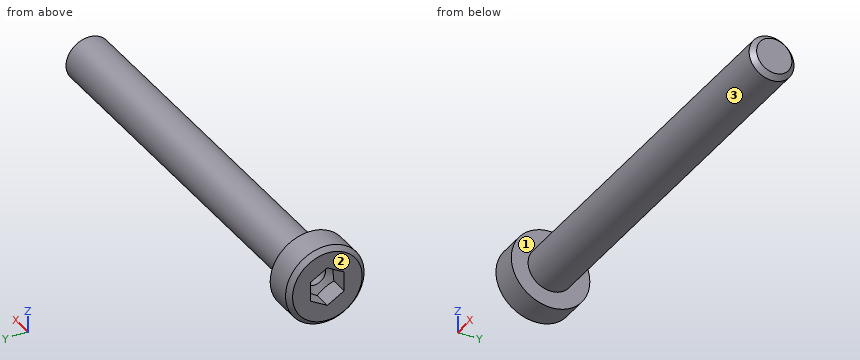
Autodesk Inventor part; units mm, degrees
ref_plane "Work Plane1" through (17.5, 0, 0) normal (0, 0.5, 0.866) x (1, 0, 0)
ref_plane "YZ Plane" through (0, 0, 0) normal (1, 0, 0) x (0, 1, 0)
ref_plane "XZ Plane" through (0, 0, 0) normal (0, 1, 0) x (-1, 0, 0)
sketch "Sketch1" plane through (0, 0, 0) normal (0, 0, 1) x (1, 0, 0)
  line L0 (1.0774, 0) -> (35, 0)
  line L1 (35, 0) -> (35, 2)
  line L2 (35, 2) -> (0, 2)
  line L3 (0, 2) -> (0, 3.5)
  line L4 (0, 3.5) -> (-2.8, 3.5)
  line L5 (-2.8, 3.5) -> (-2.8, 1.7321)
  line L6 (-2.8, 1.7321) -> (-1.2, 1.7321)
  line L7 (-1.2, 1.7321) -> (-0.7774, 1)
  line L8 (-10.36, 0) -> (42.56, 0)
  line L9 (0, -0.7) -> (0, 4.2)
  line L10 (-0.7774, 1) -> (0.5, 1)
  line L11 (0.5, 1) -> (1.0774, 0)
  line L12 (-2.8, 1.7321) -> (-2.8, 0) construction
  line L13 (-2.8, 3.1) -> (-2.4, 3.5)
  dimension "d0" = 2.8
  dimension "d1" = 1.6
  dimension "d2" = 60
  dimension "d3" = 4
  dimension "d4" = 3.4641
  dimension "d5" = 7
  dimension "d15" = 3.3
  dimension "d16" = 2
  dimension "d17" = 35
  dimension "d32" = 45
  dimension "d33" = 0.4
revolve "Body" add sketch "Sketch1" angle 360 about axis through (1.0774, 0, 0) along (1, 0, 0) contours L11 L10 L9 L2 L1 L0 | L10 L7 L6 L5 L13 L4 L3 L9 | L13 L5 L4
revolve "Chamfer2" cut sketch "Sketch1" angle 360 about axis through (-10, 0, 0) along (1, 0, 0) contours L13 L5 L4
sketch "Sketch2" plane through (-2.8, 0, 0) normal (-1, 0, 0) x (0, 0, 1)
  circle A0 centre (0, 0) radius 1.7321
  line L0 (0, -4.9) -> (0, 4.9)
  line L1 (-4.9, 0) -> (4.9, 0)
  line L2 (1.7321, 0) -> (0.866, -1.5)
  line L3 (0.866, -1.5) -> (-0.866, -1.5)
  line L4 (-0.866, -1.5) -> (-1.7321, 0)
  line L5 (-1.7321, 0) -> (-0.866, 1.5)
  line L6 (-0.866, 1.5) -> (0.866, 1.5)
  line L7 (0.866, 1.5) -> (1.7321, 0)
extrude "Slot" add sketch "Sketch2" against normal up to next contours L7 A0 | A0 L2 | L6 L0 A0 | A0 L0 L3 | L0 L6 A0 | A0 L3 L0 | L4 A0 | A0 L5
thread "Thread"
chamfer "Chamfer1" distance 0.4294 distance2 0.4294 1 edges at (35, -2, 0) measured on face at (35, 0.0262, -0.4421)
ref_plane "Work Plane1" through (17.5, 0, 0) normal (0, 0.5, 0.866) x (1, 0, 0)
equation "\"d0\" = KOH"
equation "\"d1\" = INTI"
equation "\"d3\" = GD"
equation "\"d4\" = 1.1547 * SW"
equation "\"d5\" = KOD"
equation "\"d15\" = INFT"
equation "\"d16\" = SDT"
equation "\"d17\" = NLG"
equation "\"d33\" = Cham"
equation "\"d7\" = GEL"
equation "\"d9\" = -0.5 * SPD + 0.5 * GD"
equation "\"d12\" = GUL"
equation "\"GD\" = NND"
equation "\"NLG\" = 35"
equation "\"GEL\" = 14"
equation "\"KOD\" = 7"
equation "\"KOH\" = 2.8"
equation "\"GUL\" = 0.61345 * PTC"
equation "\"SW\" = 3"
equation "\"INTI\" = 1.6"
equation "\"SPD\" = NND - 1.2269 * PTC"
equation "\"SDT\" = 2"
equation "\"INFT\" = 3.3"
equation "\"Cham\" = 0.4"
equation "\"TOA\" = 30deg"
equation "\"GD1\" = THREADDIA - 1.2269 * PTC"
equation "\"THREADDIA\" = 4"
equation "\"BDM\" = NND"
equation "\"FAWI\" = 45deg"
equation "\"RR\" = 0.1 * NND"
equation "\"PTC\" = 0.7"
equation "\"NND\" = 4"
equation "\"FAWI1\" = 45deg"
equation "\"GAL\" = 0.61345 * PTC"
equation "\"E0\" = 1.155 * SW"
properties part number "DIN 6912 - M4 x 35" material "Steel, Mild"
Design review of the part built by this model. Coordinates are the model's own, in mm. Face numbers are marked on the shaded views. Coordinates: 2 decimals unless noted, no trailing zeros. Loops run counter-clockwise (first coordinate to the right, second up) from the corner with the lowest first, then second, coordinate; pieces in that order, holes last.
Q1. To check wall thickness, follow line 1 (Z direction, x = 0.2, y = 0); line 2 (Z direction, x = -0.2, y = 0); line 3 (Z direction, x = 7.5, y = 0). State the ranges of each line that lie inside material, in increasing order.
Reported:
line 1: z = -2 to -1, 1 to 2
line 2: z = -3.5 to -1, 1 to 3.5
line 3: z = -2 to 2
Q2. We need section A-A on x = 23. State the section outline as (y, z) points.
Reported:
outline: circle Ø4 at (0, 0)
Q3. For pin 1 (2 mm diameter, centred on y = -1, z = -2.5, fed in from +X); pin 2 (4 mm diameter, centred on x = 9, z = 0.5, fed in from -Y); pin 3 (3 mm diameter, centred on x = 17, z = 2.5, fed in from -Y), all flat-tipped, find the tip position at first contact; note any pin that passes through.
Reported:
pin 1: stops at x = 34.88
pin 2: stops at y = -2
pin 3: stops at y = -1.73
Q4. The part is to be moulded in two halves that separate along X. For the marked faces 1, 2 and 3, say which applies: +X half, -X half, draft (parallel to the pull), parting line (faces both ways), or undercut.
Reported:
face 1: +X half
face 2: -X half
face 3: draft
